The model under review builds one solid part; all positions refer to its coordinate system, in mm. A direction names the side the tool comes from. Give positions to 0.01 mm unless a question says otherwise; leave off trailing zeros. Order: outer loops, then holes, each group sorted by start corner. A loop starts at its lowest first (then second) coordinate and runs counter-clockwise, first axis right, second up. Notation, with made-up numbers: (-8, -16) - (37, -16) arc R8 cw to (37, -5) - close; hole circle Ø2 at (54.5, -22). An arc over 180 degrees is marked (long way). Use a Markdown table: item, result. Add a question column.
```python
from build123d import *

# Parameters (mm, degrees)
F0_R     = 9.8044
F1_DEPTH = 5.842
F3_DEPTH = 5.843
F4_R     = 14.0335
F4_R_2   = 9.8044
F5_DEPTH = 11.049
F6_R     = 11.2395
F6_R_2   = 9.8044
F7_DEPTH = 25.4


# Not quite as in the source:
# - a pattern or mirror of a feature is missing from the dataset's text; its kind, count and spacing are read off the source's solid


with BuildPart() as f1:
    # F0 (on Front) → F1 (new body)
    with BuildSketch(Plane.XZ):
        with BuildLine():
            Line((25.6843695652, 6.1756276837), (9.7403478261, 15.9266187632))
            ThreePointArc((9.7403478261, 15.9266187632), (0, 18.669), (-9.7403478261, 15.9266187632))
            Line((-9.7403478261, 15.9266187632), (-25.6843695652, 6.1756276837))
            ThreePointArc((-25.6843695652, 6.1756276837), (-29.1465, 0), (-25.6843695652, -6.1756276837))
            Line((-25.6843695652, -6.1756276837), (-9.7403478261, -15.9266187632))
            ThreePointArc((-9.7403478261, -15.9266187632), (0, -18.669), (9.7403478261, -15.9266187632))
            Line((9.7403478261, -15.9266187632), (25.6843695652, -6.1756276837))
            ThreePointArc((25.6843695652, -6.1756276837), (29.1465, 0), (25.6843695652, 6.1756276837))
        make_face()
        Circle(F0_R, mode=Mode.SUBTRACT)
    extrude(amount=F1_DEPTH)

    # F2 (on face) → F3 (cut, through all)
    with BuildSketch(Plane.XZ.offset(5.842)):
        with BuildLine():
            ThreePointArc((-23.1775, 3.5814), (-26.7589, 0), (-23.1775, -3.5814))
            Line((-23.1775, -3.5814), (-20.6375, -3.5814))
            ThreePointArc((-20.6375, -3.5814), (-17.0561, 0), (-20.6375, 3.5814))
            Line((-20.6375, 3.5814), (-23.1775, 3.5814))
        make_face()
    f3 = extrude(amount=-F3_DEPTH, mode=Mode.SUBTRACT)

    # F3_copies: F3 across plane
    add(f3.mirror(Plane(origin=(0, 0, 0), x_dir=(0, 0, 1), z_dir=(1, 0, 0))), mode=Mode.SUBTRACT)

    # F4 (on face) → F5 (join)
    with BuildSketch(Plane.XZ.offset(5.842)):
        Circle(F4_R)
        Circle(F4_R_2, mode=Mode.SUBTRACT)
    extrude(amount=F5_DEPTH)

    # F6 (on face) → F7 (join)
    with BuildSketch(Plane(origin=(0, 0, 0), x_dir=(-1, 0, 0), z_dir=(0, 1, 0))):
        Circle(F6_R)
        Circle(F6_R_2, mode=Mode.SUBTRACT)
    extrude(amount=F7_DEPTH)


solid = f1.part
```
Q1. Wall thickness on probe 1 along Z at (x, y) = (0, 15); probe 2 along Z at (x, y) = (0, -7); probe 3 along X at (y, z) = (-3, 1): over which ranges is each line inside the solid? List them lowest first.
Q2. We need section B-B (z = 9). Write out the cut boundary in (x, y).
Q3. Clearance check with flat-ended pins moving along their axes: P1, Ø2, axis at x = 22, y = -3.5, coming from the -Z side; P2, Ø4, axis at y = 3.5, z = 6.5, coming from the -X side; P3, Ø3, axis at x = -11, y = -2.5, coming from the +Z side. State where each tip first meets the part, or that it passes through.
Q4. Draft analysis for pull direction X (two halves, no side actions). For faces 5 (the flat face through (-22, -3, 3.581)), 6 (the flat face through (-1, 25.4, 10)), 7 (the cylindrical face through (26.76, -2.96, 0.08)), 8 (the flat face through (-17.824, -2.88, -10.983)), state which applies: pulls with the +X half, pulls with the -X half, needs draft (parallel to the pull), parting line crosses it, or undercut.
Q5. We need section D-D (y = 8). Write out the cut boundary in (x, z).
Q6. We need section C-C (z = 0). Write out the cut boundary in (x, y).
Q7. Machinability: for faces 1 (the flat face through (17.6, -2.88, -11.12)), 2 (the flat face through (0, 0, 13)), 3 (the flat face through (-22, -3, -3.581)), 4 (the cylindrical face through (-10.343, -11.289, 9.485)), which of the approach directions +Z, -Z, +X, -X, +Y, -Y give a long, thin tool a straight path to every point of the face, cutting with its end or side? Answer none if there is none.
Q8. We need section A-A (x = -24.5). Write out the cut boundary in (y, z), plus the area to 3 significant figures.
Here are the results:
| question | item | result |
|---|---|---|
| 1 | probe 1 | -11.24 to -9.8, 9.8 to 11.24 |
| 1 | probe 2 | -14.03 to -9.8, 9.8 to 14.03 |
| 1 | probe 3 | -29.08 to -26.62, -17.2 to -9.75, 9.75 to 17.2, 26.62 to 29.08 |
| 2 | outline | (-21.07, -5.84) - (-10.77, -5.84) - (-10.77, -16.89) - (-3.89, -16.89) - (-3.89, 25.4) - (-6.73, 25.4) - (-6.73, 0) - (-21.07, 0) - close; (3.89, -16.89) - (10.77, -16.89) - (10.77, -5.84) - (21.07, -5.84) - (21.07, 0) - (6.73, 0) - (6.73, 25.4) - (3.89, 25.4) - close |
| 3 | P1 | z = -9.04 |
| 3 | P2 | x = -10.3 |
| 3 | P3 | z = 16.07 |
| 4 | face 5 | undercut |
| 4 | face 6 | needs draft |
| 4 | face 7 | undercut |
| 4 | face 8 | pulls with the -X half |
| 5 | outline | circle Ø22.48 at (0, 0); hole circle Ø19.61 at (0, 0) |
| 6 | outline | (-29.15, -5.84) - (-26.76, -5.84) - (-26.76, 0) - (-29.15, 0) - close; (-17.06, -5.84) - (-14.03, -5.84) - (-14.03, -16.89) - (-9.8, -16.89) - (-9.8, 25.4) - (-11.24, 25.4) - (-11.24, 0) - (-17.06, 0) - close; (9.8, -16.89) - (14.03, -16.89) - (14.03, -5.84) - (17.06, -5.84) - (17.06, 0) - (11.24, 0) - (11.24, 25.4) - (9.8, 25.4) - close; (26.76, -5.84) - (29.15, -5.84) - (29.15, 0) - (26.76, 0) - close |
| 7 | face 1 | -Z, +X, +Y, -Y |
| 7 | face 2 | +Y |
| 7 | face 3 | +Y, -Y |
| 7 | face 4 | -Y |
| 8 | outline | (-5.84, -6.9) - (0, -6.9) - (0, -3.33) - (-5.84, -3.33) - close; (-5.84, 3.33) - (0, 3.33) - (0, 6.9) - (-5.84, 6.9) - close |
| 8 | area | 41.7 mm2 |
